Build history of the part. All positions in model axes, mm. A direction names the side the tool comes from. Give positions to 0.01 mm unless a question says otherwise; leave off trailing zeros. Order: outer loops, then holes, each group sorted by start corner. A loop starts at its lowest first (then second) coordinate and runs counter-clockwise, first axis right, second up. Notation, with made-up numbers: (-29, 70.25) -> (22, 70.25) arc R23 ccw to (22, 78.25) -> close; hole circle Ø9 at (-39.75, -37.5). An arc over 180 degrees is marked (long way). One line per item, written item: value. Start each with the question number.
(1) Pin check, flat tips, straight feed: pin 1 (1 mm diameter, centred on x = 4, y = 5, fed in from +Z); pin 2 (3 mm diameter, centred on x = 3, y = 6.5, fed in from -Z). Stop position of each tip, or through.
(2) Which spindle directions (+Z, -Z, +X, -X, +Y, -Y) get a long thin tool onto all of the face, cutting with end or side? Do faces 5 (the flat face through (3, 2, 0)), 6 (the flat face through (4.4, -0.5, -8)). Say none if no direction does.
(3) Saw through at A-A on z = 0.25. Give the cut face in (x, y), plus the area to 3 significant figures.
(4) Two-plate mould, pull along Y, no slides. Class faces 1 (the flat face through (0, -0.2, -1.8)), 2 (the cylindrical face through (2.9, 2.8, 0.5)), 3 (the flat face through (4, -1, -3)), 4 (the cylindrical face through (7.797, 6.859, 0.507)): +Y half, -Y half, draft (parallel to the pull), parting line (faces both ways), or undercut.
(5) Probe line 1 (Y direction, x = 4.5, z = 0.85); line 2 (Z direction, x = 1.25, y = 5); line 3 (Y direction, x = 5.25, z = -1.5). List the from-to ranges inside material, lowest first.
(6) Saw through at D-D on x = 1.75. Give the cut face in (y, z).
(7) Saw through at B-B on x = 4.5. Give the cut face in (y, z), plus the area to 3 significant figures.
(8) Saw through at C-C on y = 3. Give the cut face in (x, z).
```python
from build123d import *

# Parameters (mm, degrees)
BOSS_EXTRUDE1_DEPTH = 9
SKETCH2_R           = 2
CUT_EXTRUDE1_DEPTH  = 10
FILLET1_R           = 4


with BuildPart() as part:
    # Sketch1 → Boss-Extrude1 (new body)
    with BuildSketch(Plane(origin=(0, 0, 0), x_dir=(0, 0, -1), z_dir=(1, 0, 0))):
        Polygon((-1, 8), (-1, -1), (8, -1), (8, 0), (0, 0), (0, 8), align=None)
    extrude(amount=BOSS_EXTRUDE1_DEPTH)

    # Sketch2 → Cut-Extrude1 (cut)
    with BuildSketch(Plane.XY.offset(1)):
        with Locations((4.5, 4)):
            Circle(SKETCH2_R)
    extrude(amount=-CUT_EXTRUDE1_DEPTH, mode=Mode.SUBTRACT)

    # Fillet1
    fillet1_edges = [part.edges().sort_by_distance(p)[0] for p in [
        (9, 8, 0.5),
        (0, 8, 0.5),
    ]]
    fillet(fillet1_edges, radius=FILLET1_R)


solid = part.part
```
Results below:
1. pin 1: passes through
1. pin 2: stops at z = 0
2. face 5: -Z, +X, -X, +Y
2. face 6: -Z, +X, -X, +Y, -Y
3. outline: (0, -1) -> (9, -1) -> (9, 4) arc R4 ccw to (5, 8) -> (4, 8) arc R4 ccw to (0, 4) -> close; hole circle Ø4 at (4.5, 4)
3. area: 61.6 mm²
4. face 1: draft
4. face 2: undercut
4. face 3: -Y half
4. face 4: +Y half
5. line 1: y = -1 to 2, 6 to 8
5. line 2: z = 0 to 1
5. line 3: y = -1 to 0
6. outline: (-1, -8) -> (0, -8) -> (0, 0) -> (7.31, 0) -> (7.31, 1) -> (-1, 1) -> close
7. outline: (-1, -8) -> (0, -8) -> (0, 0) -> (2, 0) -> (2, 1) -> (-1, 1) -> close; (6, 0) -> (8, 0) -> (8, 1) -> (6, 1) -> close
7. area: 13.0 mm²
8. outline: (0, 0) -> (2.77, 0) -> (2.77, 1) -> (0, 1) -> close; (6.23, 0) -> (9, 0) -> (9, 1) -> (6.23, 1) -> close
